Geometry check sheet. Reference: the model listing, model coordinates, mm. A direction names the side the tool comes from. Coordinates: 2 decimals unless noted, no trailing zeros. Loops run counter-clockwise (first coordinate to the right, second up) from the corner with the lowest first, then second, coordinate; pieces in that order, holes last.
from build123d import *

# Parameters (mm, degrees)
CHAMFER1_SIZE      = 0.381
CUT_EXTRUDE1_REACH = 53.301
SKETCH2_R          = 6.35
SKETCH2_R_2        = 6.223


with BuildPart() as part:
    # Sketch1 → Revolve1 (revolve)
    with BuildSketch(Plane(origin=(0, 0, 0), x_dir=(0, 0, -1), z_dir=(1, 0, 0)), mode=Mode.PRIVATE) as revolve1_sk:
        with BuildLine():
            Line((23.622, 7.2009), (24.257, 7.2009))
            ThreePointArc((24.257, 7.2009), (24.795815367, 6.977715367), (25.019, 6.4389))
            Line((25.019, 6.4389), (25.019, 3.556))
            Line((25.019, 3.556), (24.638, 3.175))
            Line((24.638, 3.175), (4.049888889, 3.175))
            Line((4.049888889, 3.175), (4.049888889, 2.413))
            Line((4.049888889, 2.413), (-25.019, 2.413))
            Line((-25.019, 2.413), (-25.019, 6.35))
            Line((-25.019, 6.35), (2.779888889, 6.35))
            Line((2.779888889, 6.35), (5.639504772, 8.001))
            Line((5.639504772, 8.001), (22.606, 8.001))
            Line((22.606, 8.001), (22.606, 6.48081))
            Line((22.606, 6.48081), (23.622, 6.48081))
            Line((23.622, 6.48081), (23.622, 7.2009))
        make_face()
    revolve(revolve1_sk.sketch.rotate(Axis((0, 0, 0), (0, 0, -1)), 90), axis=Axis((0, 0, 0), (0, 0, -1)))

    # Chamfer1
    chamfer1_edges = [part.edges().sort_by_distance(p)[0] for p in [
        (-6.35, 0, 25.019),
        (-2.413, 0, 25.019),
    ]]
    chamfer(chamfer1_edges, length=CHAMFER1_SIZE)

    # Cut-Extrude1: up to this cone (the profile starts outside it)
    cut_extrude1_end = Plane(origin=(0, 0, 25.019), z_dir=(0, 0, -1)).offset(16.800367261) * Cone(1e-06, 21.362325849, 37.000632739, align=(Align.CENTER, Align.CENTER, Align.MIN), mode=Mode.PRIVATE)
    # Sketch2 → Cut-Extrude1 (cut, up to the surface)
    with BuildSketch(Plane.XY.offset(25.019), mode=Mode.PRIVATE) as cut_extrude1_sk1:
        Circle(SKETCH2_R)
        with Locations(Location((0, 0, 0), (0, 0, 180))):
            Circle(SKETCH2_R_2, mode=Mode.SUBTRACT)
    cut_extrude1_tool1 = extrude(cut_extrude1_sk1.sketch, amount=-CUT_EXTRUDE1_REACH, mode=Mode.PRIVATE) - cut_extrude1_end
    add(cut_extrude1_tool1.solids().sort_by_distance((-6.332039, 0, 25.019))[0], mode=Mode.SUBTRACT)


solid = part.part
(1) Scan lines: L1, parallel to Y at x = 0, z = 15.75; L2, parallel to Y at x = 0, z = -12.5 (3 decimals); L3, parallel to X at y = 0.5, z = 21.5. Record each from-to range of solid material in increasing order.
Findings:
L1: y = -6.22 to -2.41, 2.41 to 6.22
L2: y = -8.001 to -3.175, 3.175 to 8.001
L3: x = -6.2 to -2.36, 2.36 to 6.2
(2) Sectioned sample at B-B on z = 0. Record the cut outline in (x, y).
Findings:
outline: circle Ø12.45 at (0, 0); hole circle Ø4.83 at (0, 0)
(3) Access from +Z, -Z, +X, -X, +Y, -Y to the whole of each face (thin tool, end or side, straight path). Record for faces 1 (the flat face through (-1, 3, 25.019)), 2 (the flat face through (3, 6, -22.606)), 3 (the cylindrical face through (-2.87, 5.52, 11.29)), 4 (the cylindrical face through (-0.94, -7.14, -23.94)), 5 (the cylindrical face through (-1.73, 7.81, -14.24)).
Findings:
face 1: +Z, +X, -X, +Y, -Y
face 2: none
face 3: +Z
face 4: -Z
face 5: +Z, -Z
(4) Draft check along Z on faces 6 (the cylindrical face through (-2.52, 1.93, -14.2)), 7 (the conical face through (2.978, 5.725, -2.959)), 8 (the flat face through (6, -3, -23.622)), 9 (the cylindrical face through (2.99, 5.75, -23.12)). Enter one of: +Z half, -Z half, draft (parallel to the pull), parting line (faces both ways), or undercut.
Findings:
face 6: draft
face 7: +Z half
face 8: undercut
face 9: undercut
(5) Sectioned sample at A-A on z = -7.5. Record the cut outline in (x, y) (3 decimals).
Findings:
outline: circle Ø16.002 at (0, 0); hole circle Ø6.35 at (0, 0)
(6) Gauge pin test, flat ends, axial feed: pin 1 Ø4 at (y, z) = (4, -3.5) entering from +X; pin 2 Ø4 at (x, z) = (-2.5, 3.5) entering from -Y; pin 3 Ø4.5 at (x, y) = (0, 0) entering from +Z; pin 4 Ø5 at (y, z) = (0.5, 18) entering from +X. Record the tip position at first contact, or that the pin passes through.
Findings:
pin 1: stops at x = 7.17
pin 2: stops at y = -6.2
pin 3: passes through
pin 4: stops at x = 6.22
